Source: CAD feature listing. Evaluate the final solid. Frame: model axes, mm. A direction names the side the tool comes from. Coordinates: 2 decimals unless noted, no trailing zeros. Write each loop counter-clockwise with the first axis right and the second up, starting at its lowest first coordinate (ties: lowest second). Pieces come first, ordered by that corner, then holes. Notation, with made-up numbers: (67, 49.5) - (114, 49.5) arc R26 ccw to (114, 70.5) - close; hole circle Ø10 at (-8, 10). An arc over 180 degrees is marked (long way). One line per question, with ' | ' between items.
from build123d import *

# Parameters (mm, degrees)
BOSS_EXTRUDE1_DEPTH     = 8
FILLET1_R               = 5
BOSS_EXTRUDE2_DEPTH     = 2
SKETCH3_R               = 2.05
CUT_EXTRUDE3_DEPTH      = 10
CUT_EXTRUDE3_DEPTH_BACK = 10
FILLET2_R               = 4
SKETCH6_R               = 7.5
BOSS_EXTRUDE3_DEPTH     = 6
SKETCH2_R               = 5.5
CUT_EXTRUDE4_DEPTH      = 28.386006481
CUT_EXTRUDE4_DEPTH_BACK = 3
SKETCH8_R               = 0.8
CUT_EXTRUDE5_DEPTH      = 30.928860828
FILLET3_R               = 3


with BuildPart() as part:
    # Sketch1 → Boss-Extrude1 (new body)
    with BuildSketch(Plane(origin=(0, 0, 0), x_dir=(1, 0, 0), z_dir=(0, 1, 0))):
        Polygon((0, 0), (0, 2), (26.270067987, 2), (34.518104392, -15.687971152), (32.760161227, -16.641719455), (25, 0), align=None)
    extrude(amount=BOSS_EXTRUDE1_DEPTH)

    # Fillet1
    fillet1_edges = [part.edges().sort_by_distance(p)[0] for p in [
        (26.270067987, 4, -2),
        (25, 4, 0),
    ]]
    fillet(fillet1_edges, radius=FILLET1_R)

    # Sketch5 → Boss-Extrude2 (add)
    with BuildSketch(Plane(origin=(22.344115541, 0, -10.419232191), x_dir=(-0.422618262, 0, -0.906307787), z_dir=(0.906307787, 0, -0.422618262))):
        with BuildLine():
            Line((-40.780850255, 18.736062391), (-36.467218683, 26.428860828))
            ThreePointArc((-36.467218683, 26.428860828), (-23.692308478, 4.771999965), (-36.205658542, -17.037035395))
            Line((-36.205658542, -17.037035395), (-40.049339329, -9.057253488))
            ThreePointArc((-40.049339329, -9.057253488), (-32.517126315, 5.047276383), (-40.780850255, 18.736062391))
        make_face()
    extrude(amount=-BOSS_EXTRUDE2_DEPTH)

    # Sketch3 → Cut-Extrude3 (cut, two sides)
    with BuildSketch(Plane(origin=(20.534845121, 0, -9.575555539), x_dir=(0.422618262, 0, 0.906307787), z_dir=(-0.906307787, 0, 0.422618262))) as cut_extrude3_sk:
        with Locations((28.701516689, 4)):
            Circle(SKETCH3_R)
        with Locations((34.117040182, 18.317355913)):
            Circle(SKETCH3_R)
        with Locations((48.070293023, 24.611901983)):
            Circle(SKETCH3_R)
        with Locations((62.387648936, 19.19637849)):
            Circle(SKETCH3_R)
        with Locations((68.682195005, 5.243125649)):
            Circle(SKETCH3_R)
        with Locations((63.266671512, -9.074230264)):
            Circle(SKETCH3_R)
        with Locations((49.313418672, -15.368776333)):
            Circle(SKETCH3_R)
        with Locations((34.996062759, -9.953252841)):
            Circle(SKETCH3_R)
    extrude(amount=CUT_EXTRUDE3_DEPTH, mode=Mode.SUBTRACT)
    extrude(cut_extrude3_sk.sketch, amount=-CUT_EXTRUDE3_DEPTH_BACK, mode=Mode.SUBTRACT)

    # Fillet2
    fillet2_edges = [part.edges().sort_by_distance(p)[0] for p in [
        (31.634193328, 0, 11.865238709),
        (31.549009715, 8, 11.682561863),
    ]]
    fillet(fillet2_edges, radius=FILLET2_R)

    # Sketch6 → Boss-Extrude3 (add)
    with BuildSketch(Plane(origin=(0, 0, -2), x_dir=(-1, 0, 0), z_dir=(0, 0, -1))):
        with Locations((0, 4)):
            Circle(SKETCH6_R)
    extrude(amount=-BOSS_EXTRUDE3_DEPTH)

    # Sketch2 → Cut-Extrude4 (cut, two sides)
    with BuildSketch(Plane.XY) as cut_extrude4_sk:
        with Locations((0, 4)):
            Circle(SKETCH2_R)
    extrude(amount=CUT_EXTRUDE4_DEPTH, mode=Mode.SUBTRACT)
    extrude(cut_extrude4_sk.sketch, amount=-CUT_EXTRUDE4_DEPTH_BACK, mode=Mode.SUBTRACT)

    # Sketch8 → Cut-Extrude5 (cut, through all)
    with BuildSketch(Plane(origin=(0, -3.5, 0), x_dir=(-1, 0, 0), z_dir=(0, -1, 0))):
        with Locations((0, -1.034043254)):
            Circle(SKETCH8_R)
    extrude(amount=-CUT_EXTRUDE5_DEPTH, mode=Mode.SUBTRACT)

    # Fillet3
    fillet3_edges = [part.edges().sort_by_distance(p)[0] for p in [
        (7.5, 4, 0),
    ]]
    fillet(fillet3_edges, radius=FILLET3_R)


solid = part.part
Item 1: Cut plane A-A on x = 0. Return loops of the section in (y, z), and give its area (3 significant figures).
Check sheet entries:
outline: (-3.5, -2) - (-1.5, -2) - (-1.5, 0.23) - (-3.5, 0.23) - close; (-3.5, 1.83) - (-1.5, 1.83) - (-1.5, 4) - (-3.5, 4) - close; (9.5, -2) - (11.5, -2) - (11.5, 0.23) - (9.5, 0.23) - close; (9.5, 1.83) - (11.5, 1.83) - (11.5, 4) - (9.5, 4) - close | area: 17.6 mm²
Item 2: Cut plane C-C on x = 14. Return loops of the section in (y, z), and give its area (3 significant figures).
Check sheet entries:
outline: (0, -2) - (8, -2) - (8, 0) - (0, 0) - close | area: 16.0 mm²
Item 3: Ray query, line 1 along Z through (x, y) = (0, -2.05); line 2 along X through (y, z) = (4, 2.75); line 3 along X through (y, z) = (-2, 0.5). Return the intervals inside material, ascending. Write a range as [from, to].
Check sheet entries:
line 1: [-2, 0.23], [1.83, 4] | line 2: [-7.5, -5.5], [5.5, 7.51], [26.28, 28.49] | line 3: [-4.5, -0.6], [0.6, 4.5]
Item 4: Pin query (flat end, axial travel): pin 1 Ø1.5 at (x, z) = (3, 2.5) entering from -Y; pin 2 Ø8 at (x, y) = (27.5, 12.5) entering from -Z; pin 3 Ø2 at (y, z) = (10, 19) entering from +X. Return the tip coordinate at first contact, or that it passes through.
Check sheet entries:
pin 1: y = -3.15 | pin 2: z = 12.37 | pin 3: x = 36.51
Item 5: Cut plane D-D on y = 14. Return loops of the section in (x, z), and give its area (3 significant figures).
Check sheet entries:
outline: (31.32, 13.55) - (33.13, 12.71) - (37.35, 21.76) - (35.54, 22.61) - close | area: 20.0 mm²
Item 6: Cut plane B-B on y = 4. State how many separate pieces and enclosed holes the cut face has, and give its area (3 significant figures).
Check sheet entries:
separate pieces: 3 | enclosed holes: 0 | area: 99.1 mm²
Item 7: Mould query, pull axis Z, two halves, no side actions, for faces 4 (the face through (25.738, 4.056, -1.238)), 5 (the face through (19.7, 8, -0.2)), 6 (the face through (35.656, 16.316, 20.527)). Classes: pulls with the +Z half, pulls with the -Z half, needs draft (parallel to the pull), parting line crosses it, or undercut.
Check sheet entries:
face 4: pulls with the -Z half | face 5: needs draft | face 6: undercut
Item 8: Access query for faces 1 (the face through (34, 2.2, 16.9)), 2 (the face through (24.53, 4.06, 0.8)), 3 (the face through (4, 8, 4)). Directions: +Z, -Z, +X, -X, +Y, -Y. A direction counts if a zero-diameter tool reaches every point of the face in a straight line with its end or side. Return the directions, or none.
Check sheet entries:
face 1: none | face 2: +Z, +Y, -Y | face 3: +Z, -X, +Y, -Y
